Drawing for the job (mm, zero at the part's lowest x, y, z). A direction names the side the tool comes from. Coordinates: 2 decimals unless noted, no trailing zeros. Loops run counter-clockwise (first coordinate to the right, second up) from the corner with the lowest first, then second, coordinate; pieces in that order, holes last.
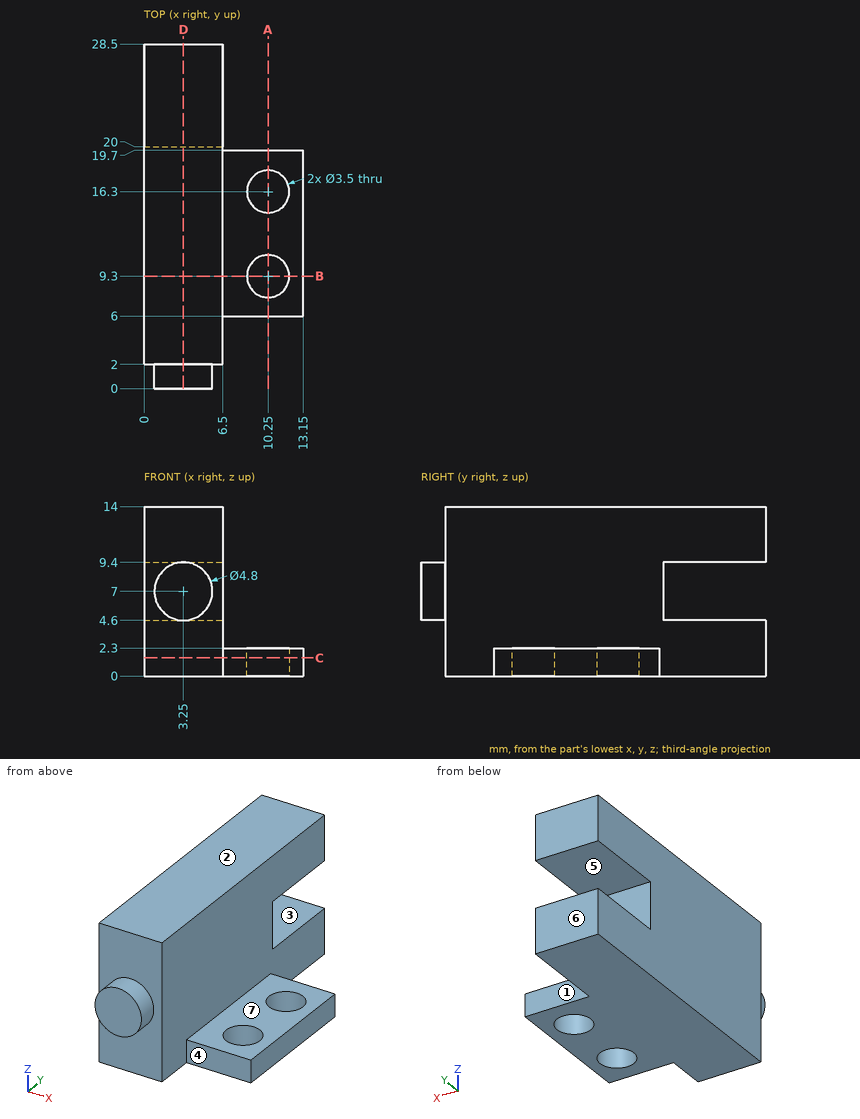
Q1. Saw through at B-B (y = 9.3). List the corners of the cut face in (x, z).
Q2. Probe line 1 (Y direction, x = 10.25, z = 1); line 2 (Y direction, x = 5, z = 12.25); line 3 (X direction, y = 19.25, z = 8). List the from-to ranges inside material, lowest first.
Q3. Saw through at D-D (x = 3.25). List the corners of the cut face in (y, z), plus the area to 3 significant figures.
Q4. Mould opens along Z. For the marked faces 1, 2 and 3 say: released by +Z, released by -Z, zero draft, split by the parting line, or undercut.
Q5. Tool access for the marked faces 4, 5, 6 and 7: list every direction of +Z, -Z, +X, -X, +Y, -Y with a clear straight run to the whole face (end or side of a thin tool).
Q6. Drop flat-ended pins along their axis: P1, Ø8, axis at y = 22.5, z = 11, coming from the +X side; P2, Ø2, axis at x = 10.25, y = 9.3, coming from the +Z side; P3, Ø1.8, axis at x = 9, z = 1, coming from the -Y side; P4, Ø5.5, axis at x = 10.25, y = 16.3, coming from the +Z side. Give the stop position or say it passes through.
Q7. Saw through at A-A (x = 10.25). List the corners of the cut face in (y, z), plus the area to 3 significant figures.
Q8. Saw through at C-C (z = 1.5). List the corners of the cut face in (x, y), plus the area to 3 significant figures.
Checked values:
1. outline: (0, 0) - (8.5, 0) - (8.5, 2.3) - (6.5, 2.3) - (6.5, 14) - (0, 14) - close; (12, 0) - (13.15, 0) - (13.15, 2.3) - (12, 2.3) - close
2. line 1: y = 6 to 7.55, 11.05 to 14.55, 18.05 to 19.7
2. line 2: y = 2 to 28.5
2. line 3: x = 0 to 6.5
3. outline: (0, 4.6) - (2, 4.6) - (2, 0) - (28.5, 0) - (28.5, 4.6) - (20, 4.6) - (20, 9.4) - (28.5, 9.4) - (28.5, 14) - (2, 14) - (2, 9.4) - (0, 9.4) - close
3. area: 340 mm2
4. face 1: zero draft
4. face 2: released by +Z
4. face 3: undercut
5. face 4: +Z, -Z, +X, -Y
5. face 5: +X, -X, +Y
5. face 6: +Z, -Z, +X, -X, +Y
5. face 7: +Z, +X, +Y, -Y
6. P1: stops at x = 6.5
6. P2: passes through
6. P3: stops at y = 6
6. P4: stops at z = 2.3
7. outline: (6, 0) - (7.55, 0) - (7.55, 2.3) - (6, 2.3) - close; (11.05, 0) - (14.55, 0) - (14.55, 2.3) - (11.05, 2.3) - close; (18.05, 0) - (19.7, 0) - (19.7, 2.3) - (18.05, 2.3) - close
7. area: 15.4 mm2
8. outline: (0, 2) - (6.5, 2) - (6.5, 6) - (13.15, 6) - (13.15, 19.7) - (6.5, 19.7) - (6.5, 28.5) - (0, 28.5) - close; hole circle Ø3.5 at (10.25, 9.3); hole circle Ø3.5 at (10.25, 16.3)
8. area: 244 mm2
